from build123d import *

# Parameters (mm, degrees)
SZKIC3_W                    = 50
SZKIC3_H                    = 50
SZKIC3_R                    = 18
SZKIC3_R_2                  = 8.25
DODANIE_WYCI_GNI_CIE2_DEPTH = 3
SZKIC4_W                    = 50
SZKIC4_H                    = 50
SZKIC4_W_2                  = 46
SZKIC4_H_2                  = 46
DODANIE_WYCI_GNI_CIE3_DEPTH = 22
ZAOKR_GLENIE1_R             = 2


with BuildPart() as part:
    # Szkic3 → Dodanie-wyciągnięcie2 (new body)
    with BuildSketch(Plane(origin=(0, 0, 0), x_dir=(1, 0, 0), z_dir=(0, 1, 0))):
        Rectangle(SZKIC3_W, SZKIC3_H)
        with Locations((4, 4)):
            Circle(SZKIC3_R, mode=Mode.SUBTRACT)
        with Locations((4, 4)):
            Circle(SZKIC3_R)
        with Locations((4, 4)):
            Circle(SZKIC3_R_2, mode=Mode.SUBTRACT)
    extrude(amount=DODANIE_WYCI_GNI_CIE2_DEPTH)

    # Szkic4 → Dodanie-wyciągnięcie3 (add)
    with BuildSketch(Plane(origin=(0, 3, 0), x_dir=(1, 0, 0), z_dir=(0, 1, 0))):
        Rectangle(SZKIC4_W, SZKIC4_H)
        Rectangle(SZKIC4_W_2, SZKIC4_H_2, mode=Mode.SUBTRACT)
    extrude(amount=DODANIE_WYCI_GNI_CIE3_DEPTH)

    # Zaokrąglenie1
    zaokr_glenie1_edges = [part.edges().sort_by_distance(p)[0] for p in [
        (-25, 12.5, 25),
        (-25, 12.5, -25),
        (25, 12.5, -25),
        (25, 12.5, 25),
        (23, 14, -23),
        (-23, 14, -23),
        (-23, 14, 23),
        (23, 14, 23),
    ]]
    fillet(zaokr_glenie1_edges, radius=ZAOKR_GLENIE1_R)


solid = part.part
The listing builds one solid part. Answer for the finished solid, in the listing's coordinates (mm). A direction names the side the tool comes from. Coordinates: 2 decimals unless noted, no trailing zeros. Order: outer loops, then holes, each group sorted by start corner. A loop starts at its lowest first (then second) coordinate and runs counter-clockwise, first axis right, second up.
Q1. A cutting plane is placed at A-A, the plane y = 11.5. Write down the section's boundary in (x, z).
Q2. A cutting plane is placed at C-C, the plane x = 4. Write down the section's boundary in (y, z), and give its area (4 significant figures).
Q3. A cutting plane is placed at B-B, the plane z = -4. Write down the section's boundary in (x, y).
Q4. For a pull along X with two mould halves and no side action, classify faces 3 (the face through (-6, 0, 0)), 4 (the face through (0, 14, -23)), 5 (the face through (-24.43, 12.68, 24.4)) as pulls with the +X half, pulls with the -X half, needs draft (parallel to the pull), parting line crosses it, or undercut.
Q5. A cutting plane is placed at D-D, the plane z = 7.5. Write down the section's boundary in (x, y), and give its area (3 significant figures).
Q6. Which of the six approach directions +Z, -Z, +X, -X, +Y, -Y give full straight-line access (tool end or side, diameter ignored) to faces 1 (the face through (-22.4, 14.15, 22.43)), 2 (the face through (24.4, 12.68, 24.43))?
Q7. Consider line 1 (Z direction, x = -2.5, y = 15); line 2 (Z direction, x = 4, y = 0.8). Determine where each line is inside the solid, lowest interval first.
Answers follow:
1. outline: (-25, -23) arc R2 ccw to (-23, -25) - (23, -25) arc R2 ccw to (25, -23) - (25, 23) arc R2 ccw to (23, 25) - (-23, 25) arc R2 ccw to (-25, 23) - close; hole (-23, -21) arc R2 ccw to (-21, -23) - (21, -23) arc R2 ccw to (23, -21) - (23, 21) arc R2 ccw to (21, 23) - (-21, 23) arc R2 ccw to (-23, 21) - close
2. outline: (0, -25) - (25, -25) - (25, -23) - (3, -23) - (3, -12.25) - (0, -12.25) - close; (0, 4.25) - (3, 4.25) - (3, 23) - (25, 23) - (25, 25) - (0, 25) - close
2. area: 188.5 mm2
3. outline: (-25, 0) - (-4.25, 0) - (-4.25, 3) - (-23, 3) - (-23, 25) - (-25, 25) - close; (12.25, 0) - (25, 0) - (25, 25) - (23, 25) - (23, 3) - (12.25, 3) - close
4. face 3: needs draft
4. face 4: undercut
4. face 5: pulls with the -X half
5. outline: (-25, 0) - (25, 0) - (25, 25) - (23, 25) - (23, 3) - (-23, 3) - (-23, 25) - (-25, 25) - close
5. area: 238 mm2
6. face 1: +Y
6. face 2: +Z, +X, +Y, -Y
7. line 1: z = -25 to -23, 23 to 25
7. line 2: z = -25 to -12.25, 4.25 to 25
